```python
from build123d import *

# Parameters (mm, degrees)
EXTRUDE_1_DEPTH              = 10
CHAMFER_1_SIZE               = 20
FILLET_1_R                   = 20
FILLET_2_R                   = 30
FILLET_3_R                   = 40
HOLE_WIZARD_M10_1_D          = 8.5
HOLE_WIZARD_M10_1_DEPTH      = 25
HOLE_WIZARD_M10_1_TIP        = 2.553657631
HOLE_WIZARD_M6_1_D           = 6.5
HOLE_WIZARD_M6_1_CBORE_D     = 11
HOLE_WIZARD_M6_1_CBORE_DEPTH = 6
HOLE_WIZARD_1_D              = 35
HOLE_WIZARD_2_D              = 16
HOLE_WIZARD_2_DEPTH          = 38
HOLE_WIZARD_M6_1_2_D         = 5
HOLE_WIZARD_M6_1_2_DEPTH     = 15
HOLE_WIZARD_M6_1_2_TIP       = 1.502151548
HOLE_WIZARD_M6_2_D           = 5
HOLE_WIZARD_M6_2_DEPTH       = 15
HOLE_WIZARD_M6_2_TIP         = 1.502151548


with BuildPart() as part:
    # 草图1 → 凸台-拉伸1 (new, symmetric)
    with BuildSketch(Plane.XY):
        with BuildLine():
            Line((0, 210), (60, 210))
            Line((60, 210), (60, 145))
            Line((60, 145), (185.093144622, 145))
            Line((185.093144622, 145), (274.574561329, 17.207293091))
            ThreePointArc((274.574561329, 17.207293091), (267.207293091, -24.574561329), (225.425438671, -17.207293091))
            Line((225.425438671, -17.207293091), (167.863272354, 65))
            Line((167.863272354, 65), (60, 65))
            Line((60, 65), (60, 0))
            Line((60, 0), (0, 0))
            Line((0, 0), (0, 210))
        make_face()
    extrude(amount=EXTRUDE_1_DEPTH, both=True)

    # 倒角1
    chamfer_1_edges = [part.edges().sort_by_distance(p)[0] for p in [
        (60, 0, 0),
        (60, 210, 0),
    ]]
    chamfer(chamfer_1_edges, length=CHAMFER_1_SIZE)

    # 圆角1
    fillet_1_edges = [part.edges().sort_by_distance(p)[0] for p in [
        (60, 145, 0),
        (60, 65, 0),
    ]]
    fillet(fillet_1_edges, radius=FILLET_1_R)

    # 圆角2
    fillet_2_edges = [part.edges().sort_by_distance(p)[0] for p in [
        (185.093144622, 145, 0),
    ]]
    fillet(fillet_2_edges, radius=FILLET_2_R)

    # 圆角3
    fillet_3_edges = [part.edges().sort_by_distance(p)[0] for p in [
        (167.863272354, 65, 0),
    ]]
    fillet(fillet_3_edges, radius=FILLET_3_R)

    # M10 螺纹孔1
    with Locations(Plane.ZY):
        with Locations((0, 195), (0, 135), (0, 75), (0, 15)):
            Hole(HOLE_WIZARD_M10_1_D / 2, depth=HOLE_WIZARD_M10_1_DEPTH)
            with Locations((0, 0, -(HOLE_WIZARD_M10_1_DEPTH + HOLE_WIZARD_M10_1_TIP / 2))):  # 118° drill point
                Cone(0, HOLE_WIZARD_M10_1_D / 2, HOLE_WIZARD_M10_1_TIP, mode=Mode.SUBTRACT)

    # Hole Wizard M6 _1 (through all)
    with Locations(Plane.XY.offset(10)):
        with Locations((70, 122.5), (70, 87.5)):
            CounterBoreHole(HOLE_WIZARD_M6_1_D / 2, HOLE_WIZARD_M6_1_CBORE_D / 2, HOLE_WIZARD_M6_1_CBORE_DEPTH)

    # 孔1 (through all)
    with Locations(Plane.XY.offset(10)):
        with Locations((150, 105)):
            Hole(HOLE_WIZARD_1_D / 2)

    # 孔2
    with Locations(Plane.XY.offset(10)):
        with Locations((250, 0)):
            Hole(HOLE_WIZARD_2_D / 2, depth=HOLE_WIZARD_2_DEPTH)

    # Hole Wizard M6 _1 2
    with Locations(Plane(origin=(0, 145, 0), x_dir=(-1, 0, 0), z_dir=(0, 1, 0))):
        with Locations((-150, 0)):
            Hole(HOLE_WIZARD_M6_1_2_D / 2, depth=HOLE_WIZARD_M6_1_2_DEPTH)
            with Locations((0, 0, -(HOLE_WIZARD_M6_1_2_DEPTH + HOLE_WIZARD_M6_1_2_TIP / 2))):  # 118° drill point
                Cone(0, HOLE_WIZARD_M6_1_2_D / 2, HOLE_WIZARD_M6_1_2_TIP, mode=Mode.SUBTRACT)

    # M6 螺纹孔2
    with Locations(Plane(origin=(192.327079244, 134.668870689, 0), x_dir=(0, 0, -1), z_dir=(0.8191520442889934, 0.573576436351044, 0))):
        with Locations((0, -143.394109088)):
            Hole(HOLE_WIZARD_M6_2_D / 2, depth=HOLE_WIZARD_M6_2_DEPTH)
            with Locations((0, 0, -(HOLE_WIZARD_M6_2_DEPTH + HOLE_WIZARD_M6_2_TIP / 2))):  # 118° drill point
                Cone(0, HOLE_WIZARD_M6_2_D / 2, HOLE_WIZARD_M6_2_TIP, mode=Mode.SUBTRACT)


solid = part.part
```
Geometry: final body of the model. Coordinates: model frame, mm. A direction names the side the tool comes from. Coordinates: 2 decimals unless noted, no trailing zeros. Order: outer loops, then holes, each group sorted by start corner. A loop starts at its lowest first (then second) coordinate and runs counter-clockwise, first axis right, second up. Notation, with made-up numbers: (34.25, 78) -> (86.25, 78) arc R16 ccw to (86.25, 109) -> close; hole circle Ø6 at (28, 15.5). An arc over 180 degrees is marked (long way). Write each question's results on one line, items separated by ' | '. Start each with the question number.
1) Mould query, pull axis X, two halves, no side actions, for faces 1 (the cylindrical face through (12.675, 199.214, 0.553)), 2 (the cylindrical face through (165.749, 60.356, -0.14)), 3 (the cylindrical face through (183.149, 141.703, -0.14)). Classes: released by +X, released by -X, zero draft, split by the parting line, or undercut.
2) Cut plane B-B, the plane x = 161. Output: boundary loops of the cut face in (y, z).
3) Set-up query: faces 4 (the flat face through (74, 123, 4)), 5 (the cylindrical face through (12.675, 139.214, 0.553)), 6 (the flat face through (60, 178, 0)). Return all of +Z, -Z, +X, -X, +Y, -Y with unobstructed straight access to the full face (end or side cutting, diameter ignored); none if empty.
4) Material intervals for line 1 along Z through (x, y) = (7.5, 15); line 2 along Y through (x, z) = (70, 5.4); line 3 along Y through (x, z) = (89, -5), sorted ascending.
5) First-contact query: pin 1 (9 mm diameter, centred on x = 70, y = 87.5, fed in from +Z); pin 2 (2 mm diameter, centred on x = 239, z = 0.5, fed in from +Y); pin 3 (8 mm diameter, centred on y = 104, z = 4, fed in from +X); pin 4 (4 mm diameter, centred on x = 70, y = 87.5, fed in from -Z). Flat tips, straight axial feed; report the tip coordinate or a pass-through.
6) Cut plane A-A, the plane x = 250. Output: boundary loops of the cut face in (y, z), and give its area (3 significant figures).
Checks:
1) face 1: zero draft | face 2: undercut | face 3: released by +X
2) outline: (62.49, -10) -> (91.39, -10) -> (91.39, 10) -> (62.49, 10) -> close; (118.61, -10) -> (145, -10) -> (145, 10) -> (118.61, 10) -> close
3) face 4: +Z | face 5: -X | face 6: +Z, -Z, +X, +Y
4) line 1: -10 to -4.25, 4.25 to 10 | line 2: 62.32 to 82, 93 to 117, 128 to 147.68 | line 3: 65 to 145
5) pin 1: z = 4 | pin 2: y = 69.44 | pin 3: x = 216.6 | pin 4: through
6) outline: (-30, -10) -> (-8, -10) -> (-8, 10) -> (-30, 10) -> close; (8, -10) -> (52.3, -10) -> (52.3, 10) -> (8, 10) -> close | area: 1,330 mm^2
